Study the drawing (mm; zero at the part's minimum x, y, z) and answer. Round coordinates to 2 decimals unless told otherwise and drop trailing zeros. Order: outer loops, then holes, each group sorted by start corner. A loop starts at its lowest first (then second) coordinate and runs counter-clockwise, first axis right, second up. Notation, with made-up numbers: M 78.25,-9 L 129.25,-9 A22 ccw 129.25,6 Z; hole C -40,4.5 d1. An arc over 180 degrees is marked long. Put each result on its own line as item: value. Start each with the question number.
1. The part is cut by section A-A (x = 57.5). Give the vertices of the cut face in (y, z), then the cut area to 3 significant figures.
2. This flat-tipped pin is pushed along its axis until it touches: pin 1 Ø0.6 at (y, z) = (0.5, 100.5) entering from -X. Where does it stop, or does it pass through?
3. The part is cut by section B-B (z = 61). Give the vertices of the cut face in (x, y).
4. The part is cut by section C-C (y = 0.55). Give the vertices of the cut face in (x, z).
5. Consider line 1 (X direction, y = 1.3, z = 113); line 2 (Z direction, x = 65, y = 1.05); line 3 (X direction, y = 0.3, z = 19). Determine where each line is inside the solid, lowest interval first.
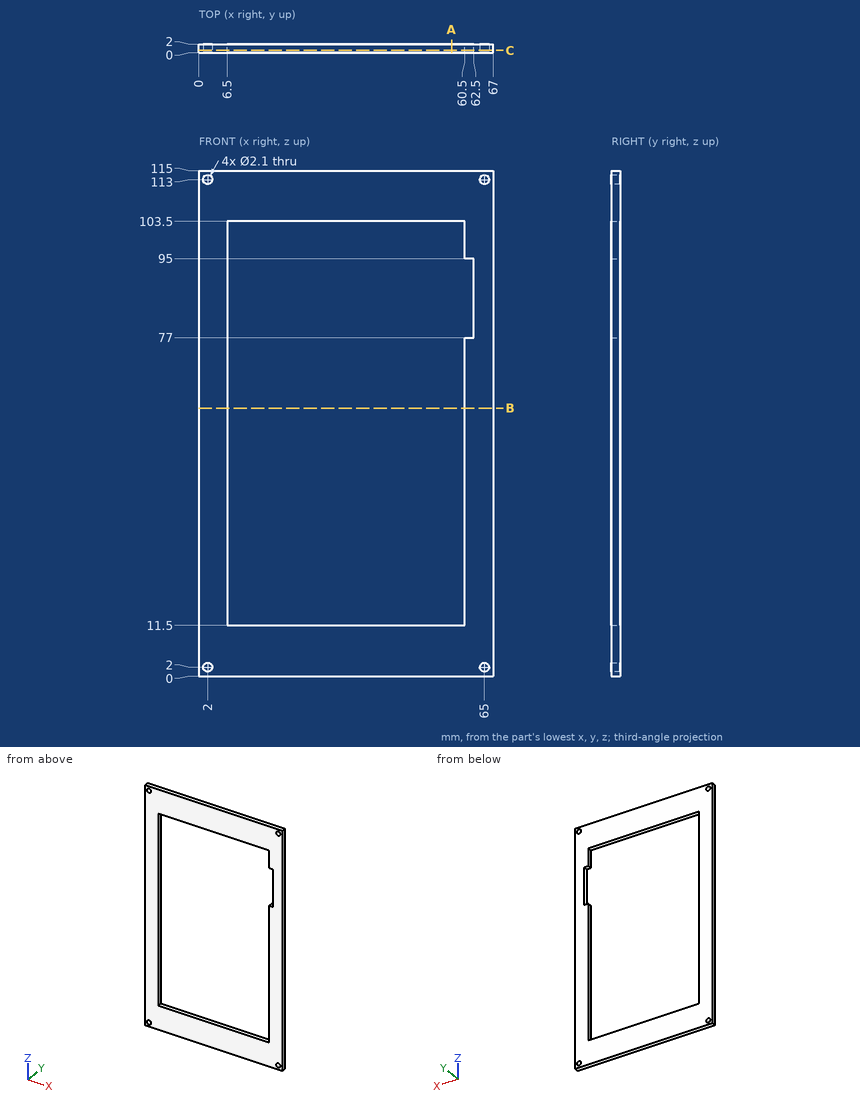
Resolved:
1. outline: M 0,0 L 2,0 L 2,11.5 L 0,11.5 Z; M 0,103.5 L 2,103.5 L 2,115 L 0,115 Z
1. area: 46.0 mm2
2. pin 1: x = 0
3. outline: M 0,0 L 6.5,0 L 6.5,2 L 0,2 Z; M 60.5,0 L 67,0 L 67,2 L 60.5,2 Z
4. outline: M 0,0 L 67,0 L 67,115 L 0,115 Z; hole C 2,2 d2.1; hole C 2,113 d2.1; hole M 6.5,11.5 L 60.5,11.5 L 60.5,77 L 62.5,77 L 62.5,95 L 60.5,95 L 60.5,103.5 L 6.5,103.5 Z; hole C 65,2 d2.1; hole C 65,113 d2.1
5. line 1: 0 to 0.95, 3.05 to 63.95, 66.05 to 67
5. line 2: 0 to 0.95, 3.05 to 111.95, 114.05 to 115
5. line 3: 0 to 6.5, 60.5 to 67
